CAD build for the part. Positions are in the model's coordinates, mm. Face numbers are marked on the shaded views. A direction names the side the tool comes from. Coordinates: 2 decimals unless noted, no trailing zeros. Order: outer loops, then holes, each group sorted by start corner. A loop starts at its lowest first (then second) coordinate and runs counter-clockwise, first axis right, second up. Notation, with made-up numbers: (86.25, -34) - (111.25, -34) arc R18 ccw to (111.25, -9) - close; hole circle Ø7 at (60, -11). An arc over 180 degrees is marked (long way). Return JSON: item names as keys, results as strings.
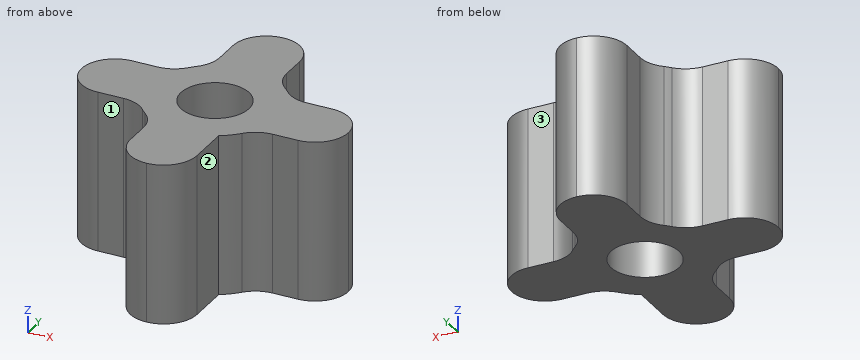
from build123d import *

# Parameters (mm, degrees)
F0_R     = 5
F0_R_2   = 2.55
F1_DEPTH = 12
F3_DEPTH = 12
F4_R     = 2.49999


# Not quite as in the source:
# - a fillet or chamfer is up to 0.001 mm smaller than in the source, because OpenCascade refuses the exact size


with BuildPart() as f1:
    # F0 (on Top) → F1 (new body)
    with BuildSketch(Plane.XY):
        Circle(F0_R)
        Circle(F0_R_2, mode=Mode.SUBTRACT)
    extrude(amount=F1_DEPTH)

    # F2 (on face) → F3 (join)
    with BuildSketch(Plane.XY.offset(12)):
        with BuildLine():
            Line((-2.5, 10), (-2.5, 4.3301270189))
            ThreePointArc((-2.5, 4.3301270189), (0, 5), (2.5, 4.3301270189))
            Line((2.5, 4.3301270189), (2.5, 10))
            Line((2.5, 10), (-2.5, 10))
        make_face()
        with BuildLine():
            Line((10, 2.5), (4.3301270189, 2.5))
            ThreePointArc((4.3301270189, 2.5), (4.8296291314, 1.2940952255), (5, 0))
            ThreePointArc((5, 0), (4.8296291314, -1.2940952255), (4.3301270189, -2.5))
            Line((4.3301270189, -2.5), (10, -2.5))
            Line((10, -2.5), (10, 2.5))
        make_face()
        with BuildLine():
            ThreePointArc((2.5, -4.3301270189), (0, -5), (-2.5, -4.3301270189))
            Line((-2.5, -4.3301270189), (-2.5, -10))
            Line((-2.5, -10), (2.5, -10))
            Line((2.5, -10), (2.5, -4.3301270189))
        make_face()
        with BuildLine():
            ThreePointArc((-4.3301270189, -2.5), (-5, 0), (-4.3301270189, 2.5))
            Line((-4.3301270189, 2.5), (-10, 2.5))
            Line((-10, 2.5), (-10, -2.5))
            Line((-10, -2.5), (-4.3301270189, -2.5))
        make_face()
    extrude(amount=-F3_DEPTH)

    # F4 (radius 2.5 in the source; OpenCascade refuses exactly that, so slightly less here)
    f4_edges = [f1.edges().sort_by_distance(p)[0] for p in [
        (2.5, -10, 6),
        (10, -2.5, 6),
        (-10, -2.5, 6),
        (-2.5, -10, 6),
        (-10, 2.5, 6),
        (-2.5, 10, 6),
        (10, 2.5, 6),
        (2.5, 10, 6),
        (2.5, 4.330127, 6),
        (4.330127, 2.5, 6),
        (4.330127, -2.5, 6),
        (-2.5, 4.330127, 6),
        (-4.330127, 2.5, 6),
        (-2.5, -4.330127, 6),
        (-4.330127, -2.5, 6),
    ]]
    fillet(f4_edges, radius=F4_R)


solid = f1.part
Item 1: Drop flat-ended pins along their axis: P1, Ø1, axis at x = -6.5, z = 6.5, coming from the -Y side; P2, Ø4.5, axis at x = 0, y = 0, coming from the +Z side; P3, Ø1.5, axis at x = 7, z = 4.5, coming from the +Y side; P4, Ø3, axis at x = -4.5, z = 6.5, coming from the +Y side. Give the stop position or say it passes through.
Findings below:
{"P1": "stops at y = -2.5", "P2": "passes through", "P3": "stops at y = 2.5", "P4": "stops at y = 4.09"}
Item 2: Band-saw the part on C-C, the plane y = 6.5. List the corners of the cut face in (x, z).
Findings below:
{"outline": "(-2.5, 0) - (2.5, 0) - (2.5, 12) - (-2.5, 12) - close"}
Item 3: Wall check: L1, parallel to Y at x = 0, z = 2.75; L2, parallel to Y at x = -7.25, z = 1.5; L3, parallel to Y at x = -1.75, z = 1.5. Give the ranges that are in metal, low to high. Write a range as [from, to].
Findings below:
{"L1": "y = [-10, -2.55], [2.55, 10]", "L2": "y = [-2.5, 2.5]", "L3": "y = [-9.29, -1.85], [1.85, 9.29]"}
Item 4: Which spindle directions (+Z, -Z, +X, -X, +Y, -Y) get a long thin tool onto all of the face, cutting with end or side? Do the marked faces 1, 2 and 3. Say none if no direction does.
Findings below:
{"face 1": "+Z, -Z, -X, -Y", "face 2": "+Z, -Z, +X, -Y", "face 3": "+Z, -Z, +X, +Y"}
Item 5: Band-saw the part on B-B, the plane x = 1.5. List the corners of the cut face in (y, z).
Findings below:
{"outline": "(-9.5, 0) - (-2.06, 0) - (-2.06, 12) - (-9.5, 12) - close; (2.06, 0) - (9.5, 0) - (9.5, 12) - (2.06, 12) - close"}
Item 6: Band-saw the part on D-D, the plane x = 4.75. List the corners of the cut face in (y, z), then the cut area to 3 significant figures.
Findings below:
{"outline": "(-2.65, 0) - (2.65, 0) - (2.65, 12) - (-2.65, 12) - close", "area": "63.5 mm²"}
